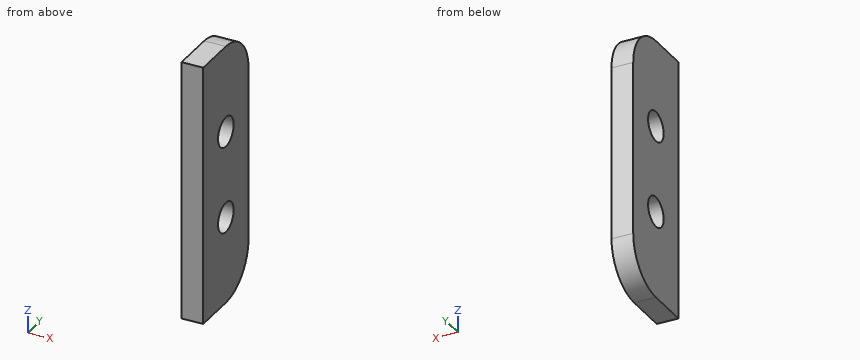
```python
from build123d import *

# Parameters (mm, degrees)
SKETCH1_W           = 48
SKETCH1_H           = 16
SKETCH1_R           = 2.75
BOSS_EXTRUDE1_DEPTH = 4
FILLET1_R           = 8


with BuildPart() as part:
    # Sketch1 → Boss-Extrude1 (new body)
    with BuildSketch(Plane(origin=(0, 0, 0), x_dir=(0, 0, -1), z_dir=(1, 0, 0))):
        Rectangle(SKETCH1_W, SKETCH1_H)
        with Locations((-8, 0)):
            Circle(SKETCH1_R, mode=Mode.SUBTRACT)
        with Locations((8, 0)):
            Circle(SKETCH1_R, mode=Mode.SUBTRACT)
    extrude(amount=BOSS_EXTRUDE1_DEPTH)

    # Fillet1
    fillet1_edges = [part.edges().sort_by_distance(p)[0] for p in [
        (2, 8, 24),
        (2, 8, -24),
    ]]
    fillet(fillet1_edges, radius=FILLET1_R)


solid = part.part
```
Verification items for the finished model (mm, model axes). Round coordinates to 2 decimals unless told otherwise and drop trailing zeros. Write each loop counter-clockwise with the first axis right and the second up, starting at its lowest first coordinate (ties: lowest second). Pieces come first, ordered by that corner, then holes. Notation, with made-up numbers: (-30.75, 38.5) -> (-2.75, 38.5) arc R24 ccw to (-2.75, 60.5) -> close; hole circle Ø4 at (-19.75, 84). An arc over 180 degrees is marked (long way). Write each question's results on one line, items separated by ' | '. Start each with the question number.
1. Cross-section at D-D (z = 20). Enter the section's corners in (x, y), then the cut area to 3 significant figures.
2. Cross-section at C-C (z = 8). Enter the section's corners in (x, y), then the cut area to 3 significant figures.
3. Depth check by flat-ended pin: P1, Ø3.5, axis at y = 0, z = 8, coming from the +X side; P2, Ø3, axis at y = -1.5, z = 8, coming from the +X side. Enter the tip coordinate at first touch or a pass-through.
4. Cross-section at B-B (y = 1.75). Enter the section's corners in (x, z), then the cut area to 3 significant figures.
5. Material ranges on probe 1 along Y at (x, z) = (2.35, -8); probe 2 along Z at (x, y) = (3.2, -2); probe 3 along Z at (x, y) = (1.1, 0.5), recorded low to high. Write a range as from..to.
6. Cross-section at A-A (x = 0.95). Enter the section's corners in (y, z), then the cut area to 3 significant figures.
Solutions:
1) outline: (0, -8) -> (4, -8) -> (4, 6.93) -> (0, 6.93) -> close | area: 59.7 mm2
2) outline: (0, -8) -> (4, -8) -> (4, -2.75) -> (0, -2.75) -> close; (0, 2.75) -> (4, 2.75) -> (4, 8) -> (0, 8) -> close | area: 42.0 mm2
3) P1: passes through | P2: stops at x = 4
4) outline: (0, -23.81) -> (4, -23.81) -> (4, -10.12) -> (0, -10.12) -> close; (0, -5.88) -> (4, -5.88) -> (4, 5.88) -> (0, 5.88) -> close; (0, 10.12) -> (4, 10.12) -> (4, 23.81) -> (0, 23.81) -> close | area: 157 mm2
5) probe 1: y = -8..-2.75, 2.75..8 | probe 2: z = -24..-9.89, -6.11..6.11, 9.89..24 | probe 3: z = -23.98..-10.7, -5.3..5.3, 10.7..23.98
6) outline: (-8, -24) -> (0, -24) arc R8 ccw to (8, -16) -> (8, 16) arc R8 ccw to (0, 24) -> (-8, 24) -> close; hole circle Ø5.5 at (0, -8); hole circle Ø5.5 at (0, 8) | area: 693 mm2
